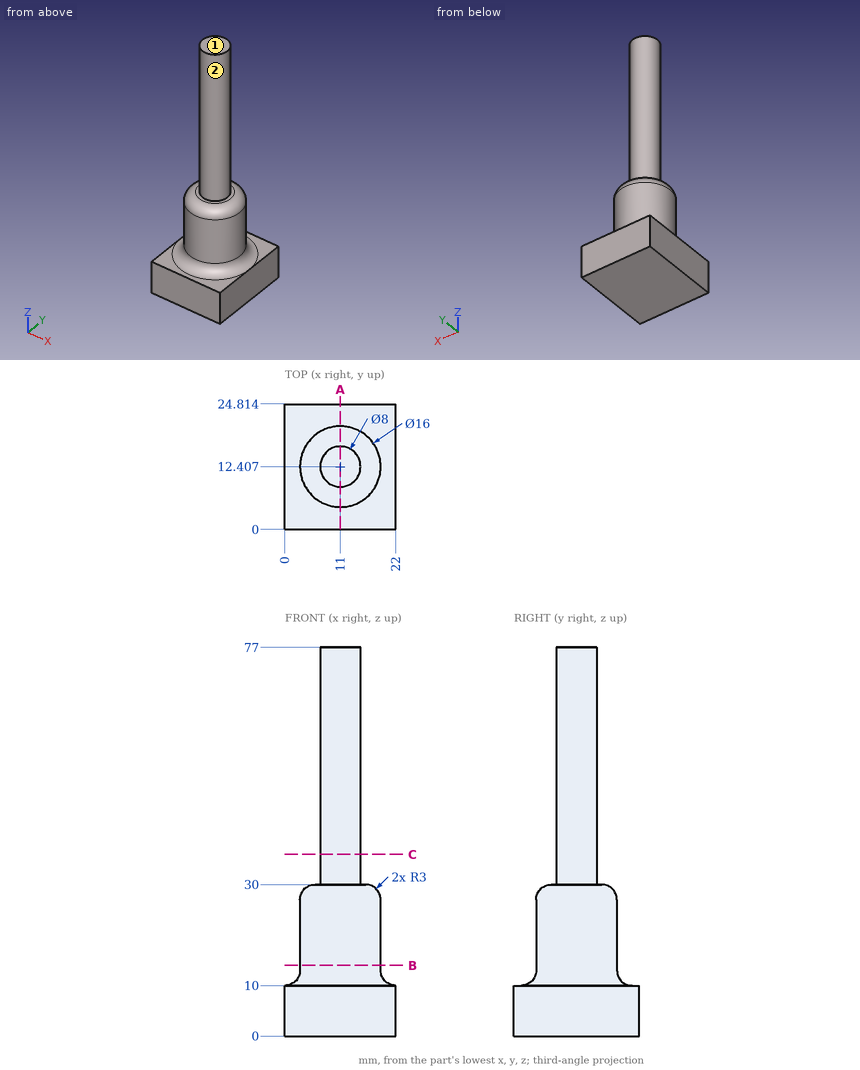
Could you check a few things on this drawing? It's one solid part, dimensions in mm from its lowest x, y, z. A direction names the side the tool comes from. Coordinates: 2 decimals unless noted, no trailing zeros. Loops run counter-clockwise (first coordinate to the right, second up) from the corner with the lowest first, then second, coordinate; pieces in that order, holes last. Notation, with made-up numbers: (89, 25.5) - (94, 25.5) arc R30 cw to (94, 56.5) - close; hole circle Ø7 at (1.5, 46). An arc over 180 degrees is marked (long way). Answer as a JSON object with one key per item and string values. Group by question number.
Item 1: On a 3-axis mill with a long thin cutter (end or side, diameter ignored), from which of +Z, -Z, +X, -X, +Y, -Y can I reach the whole of each face in a straight line? I mean the marked faces 1 and 2. Say none if no direction works.
Item 2: If we section it at B-B (z = 14): List the corners of the cut face in (x, y) for me.
Item 3: If we section it at A-A (x = 11): List the corners of the cut face in (y, z) for me.
Item 4: For pin 1 (12 mm diameter, centred on x = 4.5, z = 57, fed in from +Y); pin 2 (5 mm diameter, centred on x = 11.5, z = 26, fed in from +Y); pin 3 (5 mm diameter, centred on x = 8.5, z = 65.5, fed in from -Y); pin 4 (1 mm diameter, centred on y = 18, z = 46.5, fed in from +X), each with a flat end and sliding along its axis, tell me the tip position at first contact or that it passes through.
Item 5: If we section it at C-C (z = 36): List the corners of the cut face in (x, y) for me.
Item 6: If I drill on L1, parallel to Z at x = 16.5, y = 21.75; L2, parallel to Y at x = 11.25, z = 65; L3, parallel to X at y = 12.25, z = 32.5, over which ranges is the centre line in solid material (lowest first)? Write a range as from..to.
Returned:
{
 "1": {"face 1": "+Z, +X, -X, +Y, -Y", "face 2": "+Z"},
 "2": {"outline": "circle Ø16 at (11, 12.41)"},
 "3": {"outline": "(0, 0) - (24.81, 0) - (24.81, 10) - (23.41, 10) arc R3 cw to (20.41, 13) - (20.41, 27) arc R3 ccw to (17.41, 30) - (16.41, 30) - (16.41, 77) - (8.41, 77) - (8.41, 30) - (7.41, 30) arc R3 ccw to (4.41, 27) - (4.41, 13) arc R3 cw to (1.41, 10) - (0, 10) - close"},
 "4": {"pin 1": "stops at y = 16.38", "pin 2": "stops at y = 20.41", "pin 3": "stops at y = 8.41", "pin 4": "passes through"},
 "5": {"outline": "circle Ø8 at (11, 12.41)"},
 "6": {"L1": "z = 0..10", "L2": "y = 8.41..16.4", "L3": "x = 7..15"}
}
